Can you work these out from the model? Positions are in its coordinate system, mm. A direction names the side the tool comes from. Coordinates: 2 decimals unless noted, no trailing zeros. Loops run counter-clockwise (first coordinate to the right, second up) from the corner with the lowest first, then second, coordinate; pieces in that order, holes last.
```python
from build123d import *

# Parameters (mm, degrees)
SKETCH_R             = 2
PAD_DEPTH            = 2
PAD001_DEPTH         = 6
CHAMFER_SIZE         = 0.5
FILLET_R             = 0.99
FILLET001_R          = 1
BODY_PLACEMENT_ANGLE = 180


with BuildPart() as part:
    # Sketch → Pad (new body)
    with BuildSketch(Plane.XY):
        with BuildLine():
            ThreePointArc((7, 5), (0.981931, 11.930787), (-6.724518, 6.944444))
            ThreePointArc((-6.724518, 6.944444), (-7.708384, 0), (-6.724518, -6.944444))
            ThreePointArc((-6.724518, -6.944444), (0.981931, -11.930787), (7, -5))
            Line((7, -5), (7, 5))
        make_face()
        with Locations((0, 5)):
            Circle(SKETCH_R, mode=Mode.SUBTRACT)
        with Locations((0, -5)):
            Circle(SKETCH_R, mode=Mode.SUBTRACT)
    extrude(amount=PAD_DEPTH)

    # Sketch001 → Pad001 (join, symmetric)
    with BuildSketch(Plane.XZ):
        with BuildLine():
            Line((-6.724518, 2), (-9, 2))
            ThreePointArc((-9, 6), (-11, 4), (-9, 2))
            Line((-9, 8), (-9, 6))
            ThreePointArc((-9, 8), (-13, 4), (-9, 0))
            Line((-6.724518, 0), (-9, 0))
            Line((-6.724518, 2), (-6.724518, 0))
        make_face()
    extrude(amount=PAD001_DEPTH, both=True)

    # Chamfer
    chamfer_edges = [part.edges().sort_by_distance(p)[0] for p in [
        (-2, -5, 2),
        (-2, 5, 2),
    ]]
    chamfer(chamfer_edges, length=CHAMFER_SIZE)

    # Fillet
    fillet_edges = [part.edges().sort_by_distance(p)[0] for p in [
        (-9, 0, 8),
        (-9, 0, 6),
    ]]
    fillet(fillet_edges, radius=FILLET_R)

    # Fillet001
    fillet001_edges = [part.edges().sort_by_distance(p)[0] for p in [
        (-6.855729, 6.47346, 2),
        (0.981931, 11.930787, 2),
        (7, 0, 2),
        (0.981931, -11.930787, 2),
        (-6.855729, -6.47346, 2),
    ]]
    fillet(fillet001_edges, radius=FILLET001_R)


with BuildPart() as part_1:
    # Body placement: moved
    add(part.part.moved(Location((-26, -38, 0))).rotate(Axis((-26, -38, 0), (0, 0, 1)), BODY_PLACEMENT_ANGLE))


solid = part_1.part
```
Item 1: We'd pull the mould along Y, two halves only. Please class faces 1 (the face through (-26.923, -41.226, 0.74)), 2 (the face through (-27.12, -49.91, 0.49)), 3 (the face through (-13.044, -37.916, 3.41)): +Y half, -Y half, draft (parallel to the pull), parting line (faces both ways), or undercut.
Results are:
face 1: undercut
face 2: -Y half
face 3: draft
Item 2: I'm going to push flat-ended pins straight in: P1, Ø4.5, axis at x = -21.5, y = -35, coming from the +Z side; P2, Ø2, axis at x = -17, z = 5.5, coming from the +Y side; P3, Ø3.5, axis at x = -16, z = 6, coming from the -Y side. Where does each tip first touch, or does it pass through?
Results are:
P1: stops at z = 2
P2: stops at y = -32
P3: stops at y = -44
Item 3: On a 3-axis mill with a long thin cutter (end or side, diameter ignored), from which of +Z, -Z, +X, -X, +Y, -Y can I reach the whole of each face in a straight line? I mean faces 4 (the face through (-16.81, -37.92, 6.24)), 5 (the face through (-24, -38, 2)), 6 (the face through (-19.142, -31.533, 0.493)). Say none if no direction works.
Results are:
face 4: -X, +Y, -Y
face 5: +Z, -X, +Y, -Y
face 6: +Z, -Z, +X, +Y
Item 4: I need wall thicknesses on line 1 along Y through (x, z) = (-26, 0.65); line 2 along Z through (x, y) = (-30.5, -39.25); line 3 along X through (y, z) = (-43, 0.35). Which ranges of each line are inside material? Lowest first, please.
Results are:
line 1: y = -50 to -45, -41 to -35, -31 to -26
line 2: z = 0 to 2
line 3: x = -33 to -28, -24 to -15.36
Item 5: Suppose I cut it at B-B, the plane z = 4. Please give me the cut outline in (x, y), plus the area to 3 significant figures.
Results are:
outline: (-15, -44) - (-13, -44) - (-13, -32) - (-15, -32) - close
area: 24.0 mm2
Item 6: Suppose I cut it at C-C, the plane z = 6.5. Please give me the cut outline in (x, y), plus the area to 3 significant figures.
Results are:
outline: (-16.95, -44) - (-13.88, -44) - (-13.88, -32) - (-16.95, -32) - close
area: 36.8 mm2
